Model file for the job. Use its own axes, mm. A direction names the side the tool comes from. Give positions to 0.01 mm unless a question says otherwise; leave off trailing zeros. Loops run counter-clockwise (first coordinate to the right, second up) from the corner with the lowest first, then second, coordinate; pieces in that order, holes last. Notation, with made-up numbers: M -19,43 L 24,43 A19 cw 24,73 Z; hole C 9.25,5 d5. An arc over 180 degrees is marked long. Answer in a Markdown table with one row per item.
```python
from build123d import *

# Parameters (mm, degrees)
F0_W     = 106.6799983382
F0_H     = 73.8282129169
F1_DEPTH = 55.372
F2_W     = 87.9580117762
F2_H     = 57.2256948799
F3_DEPTH = 57.15
F4_W     = 55.8799983382
F4_H     = 30.48
F5_DEPTH = 75.438
F6_R     = 6.9922217865
F7_DEPTH = 111.252


with BuildPart() as f1:
    # F0 (on Top) → F1 (new body)
    with BuildSketch(Plane.XY):
        with Locations((2.0311586559, 1.148045063)):
            Rectangle(F0_W, F0_H)
    extrude(amount=F1_DEPTH)

    # F2 (on face) → F3 (cut)
    with BuildSketch(Plane.XY.offset(55.372)):
        with Locations((2.2077802569, 0.7948009297)):
            Rectangle(F2_W, F2_H)
    extrude(amount=-F3_DEPTH, mode=Mode.SUBTRACT)

    # F4 (on face) → F5 (cut)
    with BuildSketch(Plane.XZ.offset(35.7660613954)):
        with Locations((2.0311586559, 40.132)):
            Rectangle(F4_W, F4_H)
    extrude(amount=-F5_DEPTH, mode=Mode.SUBTRACT)

    # F6 (on face) → F7 (cut)
    with BuildSketch(Plane(origin=(-51.3088405132, 0, 0), x_dir=(0, -1, 0), z_dir=(-1, 0, 0))):
        with Locations((0, 36.295928061)):
            Circle(F6_R)
    extrude(amount=-F7_DEPTH, mode=Mode.SUBTRACT)


solid = f1.part
```
(1) Flat gauge pins, fed straight in: P1, Ø7, axis at x = 9.5, y = 34, coming from the +Z side; P2, Ø11, axis at y = 0, z = 36.3, coming from the -X side. Where does each tip first touch, or does it go through?
Established:
| item | result |
|---|---|
| P1 | stops at z = 24.89 |
| P2 | passes through |
(2) Saw through at A-A, the plane x = 42.5. Give the cut face in (y, z), and give its area (3 significant figures).
Established:
| item | result |
|---|---|
| outline | M -35.77,0 L -27.82,0 L -27.82,55.37 L -35.77,55.37 Z; M 29.41,0 L 38.06,0 L 38.06,55.37 L 29.41,55.37 Z |
| area | 919 mm2 |
(3) Which spindle directions (+Z, -Z, +X, -X, +Y, -Y) get a long thin tool onto all of the face, cutting with end or side? Do faces 4 (the flat face through (55.371, 1, 27)), 5 (the flat face through (2, 29.408, 22)), 6 (the flat face through (-25.909, 34, 40)). Say none if no direction does.
Established:
| item | result |
|---|---|
| face 4 | +Z, -Z, +X, +Y, -Y |
| face 5 | +Z, -Z |
| face 6 | +Z, +Y, -Y |
(4) Mould opens along Z. For faces 1 (the flat face through (1, -31, 0)), 2 (the flat face through (2, -32, 24.892)), 3 (the cylindrical face through (50.71, -3.76, 42.19)) say: pulls with the +Z half, pulls with the -Z half, needs draft (parallel to the pull), parting line crosses it, or undercut.
Established:
| item | result |
|---|---|
| face 1 | pulls with the -Z half |
| face 2 | pulls with the +Z half |
| face 3 | undercut |
(5) Wall check: L1, parallel to Z at x = -45, y = 0; L2, parallel to Y at x = 19.5, z = 5; L3, parallel to X at y = -24.5, z = 34.5. Give the ranges that are in metal, low to high.
Established:
| item | result |
|---|---|
| L1 | z = 0 to 29.3, 43.29 to 55.37 |
| L2 | y = -35.77 to -27.82, 29.41 to 38.06 |
| L3 | x = -51.31 to -41.77, 46.19 to 55.37 |
(6) Saw through at C-C, the plane y = 0. Give the cut face in (x, z).
Established:
| item | result |
|---|---|
| outline | M -51.31,0 L -41.77,0 L -41.77,29.3 L -51.31,29.3 Z; M -51.31,43.29 L -41.77,43.29 L -41.77,55.37 L -51.31,55.37 Z; M 46.19,0 L 55.37,0 L 55.37,29.3 L 46.19,29.3 Z; M 46.19,43.29 L 55.37,43.29 L 55.37,55.37 L 46.19,55.37 Z |
(7) Saw through at B-B, the plane z = 14. Give the cut face in (x, y), and give its area (3 significant figures).
Established:
| item | result |
|---|---|
| outline | M -51.31,-35.77 L 55.37,-35.77 L 55.37,38.06 L -51.31,38.06 Z; hole M -41.77,-27.82 L 46.19,-27.82 L 46.19,29.41 L -41.77,29.41 Z |
| area | 2,840 mm2 |
(8) Saw through at D-D, the plane z = 50.5. Give the cut face in (x, y), and give its area (3 significant figures).
Established:
| item | result |
|---|---|
| outline | M -51.31,-35.77 L -25.91,-35.77 L -25.91,-27.82 L -41.77,-27.82 L -41.77,29.41 L -25.91,29.41 L -25.91,38.06 L -51.31,38.06 Z; M 29.97,-35.77 L 55.37,-35.77 L 55.37,38.06 L 29.97,38.06 L 29.97,29.41 L 46.19,29.41 L 46.19,-27.82 L 29.97,-27.82 Z |
| area | 1,910 mm2 |
